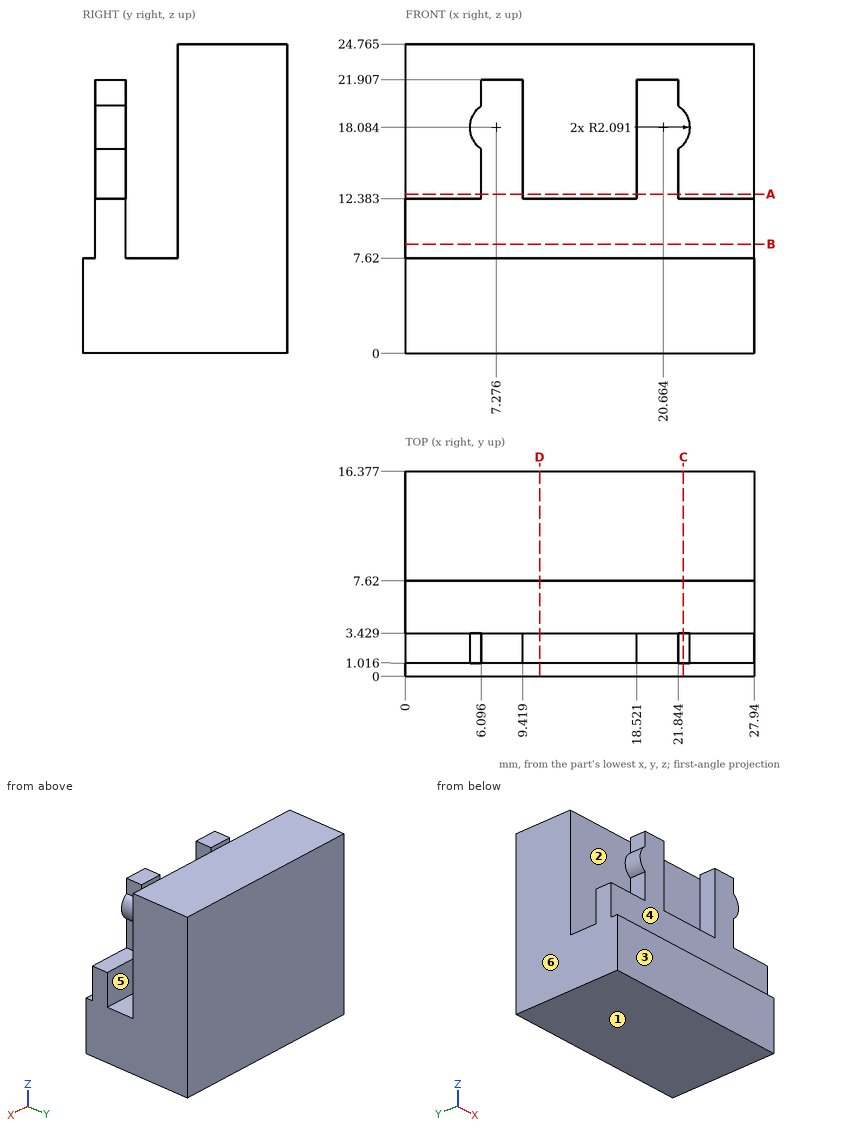
Design review of the part shown in the three views and the two pictorial views. Dimensions are in mm from the part's minimum x, y and z. A direction names the side the tool comes from. Coordinates: 2 decimals unless noted, no trailing zeros. Order: outer loops, then holes, each group sorted by start corner. A loop starts at its lowest first (then second) coordinate and runs counter-clockwise, first axis right, second up.
Item 1: For line 1 (Y direction, x = 12, z = 11.75) (1 decimal); line 2 (Z direction, x = 6.5, y = 7.5); line 3 (Y direction, x = 15.5, z = 17), list the stretches that pass through material, from the lowest coordinate up.
Item 2: For pin 1 Ø2.5 at (y, z) = (2.5, 14.5) entering from +X; pin 2 Ø1.7 at (y, z) = (2, 20.5) entering from -X; pin 3 Ø2 at (x, y) = (25, 2) entering from +Z, all flat-tipped, find the tip position at first contact; note any pin that passes through.
Item 3: For the marked faces 4, 5 and 6, list the 3-axis set-ups (+Z, -Z, +X, -X, +Y, -Y) from which the entire face can be reached by the end or side of a thin tool; tool diameter is ignored.
Item 4: Take a section at D-D, the plane x = 10.75. Write out the cut boundary in (y, z) (1 decimal).
Item 5: Take a section at B-B, the plane z = 8.75. Write out the cut boundary in (x, y) (1 decimal).
Item 6: The part is to be moulded in two halves that separate along Y. For the marked faces 1, 2 and 3, say which applies: pulls with the +Y half, pulls with the -Y half, needs draft (parallel to the pull), parting line crosses it, or undercut.
Item 7: Take a section at C-C, the plane x = 22.25. Write out the cut boundary in (y, z) (1 decimal).
Item 8: Take a section at A-A, the plane z = 12.75. Write out the cut boundary in (x, y) (1 decimal).
The answers:
1. line 1: y = 1 to 3.4, 7.6 to 16.4
1. line 2: z = 0 to 7.62
1. line 3: y = 7.62 to 16.38
2. pin 1: stops at x = 21.84
2. pin 2: stops at x = 5.89
2. pin 3: stops at z = 12.38
3. face 4: +Z, +X, -X, -Y
3. face 5: +Z, +X, -X
3. face 6: +Z, -Z, -X, +Y, -Y
4. outline: (0, 0) - (16.4, 0) - (16.4, 24.8) - (7.6, 24.8) - (7.6, 7.6) - (3.4, 7.6) - (3.4, 12.4) - (1, 12.4) - (1, 7.6) - (0, 7.6) - close
5. outline: (0, 1) - (27.9, 1) - (27.9, 3.4) - (0, 3.4) - close; (0, 7.6) - (27.9, 7.6) - (27.9, 16.4) - (0, 16.4) - close
6. face 1: needs draft
6. face 2: undercut
6. face 3: pulls with the -Y half
7. outline: (0, 0) - (16.4, 0) - (16.4, 24.8) - (7.6, 24.8) - (7.6, 7.6) - (3.4, 7.6) - (3.4, 12.4) - (1, 12.4) - (1, 7.6) - (0, 7.6) - close; (1, 16.7) - (3.4, 16.7) - (3.4, 19.4) - (1, 19.4) - close
8. outline: (0, 7.6) - (27.9, 7.6) - (27.9, 16.4) - (0, 16.4) - close; (6.1, 1) - (9.4, 1) - (9.4, 3.4) - (6.1, 3.4) - close; (18.5, 1) - (21.8, 1) - (21.8, 3.4) - (18.5, 3.4) - close
